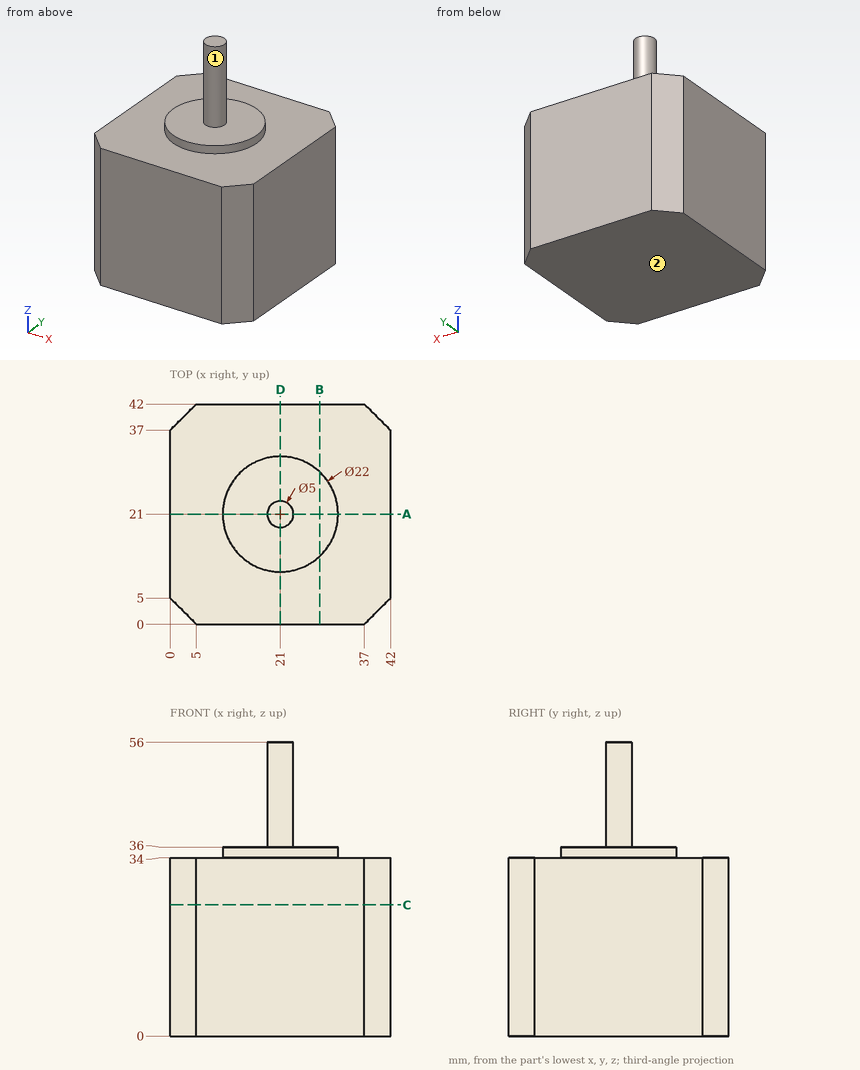
Study the drawing (mm; zero at the part's minimum x, y, z) and answer. A direction names the side the tool comes from. Give positions to 0.01 mm unless a question says otherwise; leave off trailing zeros. Write each loop counter-clockwise with the first axis right and the second up, starting at its lowest first coordinate (ties: lowest second). Pieces come first, ordered by that corner, then holes. Notation, with made-up numbers: (39, -0.75) -> (77, -0.75) arc R27 cw to (77, 31.25) -> close; hole circle Ø2 at (23.5, 23.25). An arc over 180 degrees is marked (long way). Answer as a JSON object with one key per item and string values. Group by question number.
1) Find section C-C (z = 25). Write down the section's boundary in (x, y), and give its area (3 significant figures).
2) Find section A-A (y = 21). Write down the section's boundary in (x, z).
3) Consider L1, parallel to Z at x = 31, y = 7; L2, parallel to Z at x = 25, y = 14.5. Determine where each line is inside the solid, lowest interval first. Write a range as from..to.
4) A tool of negligible diameter and unlimited length cuts with its end or side. For the marked faces 1 and 2, from which of +Z, -Z, +X, -X, +Y, -Y can it reach the whole face along a straight path? Write none if from no direction.
5) Find section B-B (x = 28.5). Write down the section's boundary in (y, z), and give its area (3 significant figures).
6) Each of these flat-tipped pins is pushed along its axis until it touches: P1, Ø6.5, axis at x = 23, y = 16, coming from the +Z side; P2, Ø5, axis at x = 14.5, y = 4.5, coming from the +Z side; P3, Ø1, axis at x = 29.5, y = 18.5, coming from the +Z side. Where does it stop, or does it pass through?
Values follow:
{
 "1": {"outline": "(0, 5) -> (5, 0) -> (37, 0) -> (42, 5) -> (42, 37) -> (37, 42) -> (5, 42) -> (0, 37) -> close", "area": "1,710 mm2"},
 "2": {"outline": "(0, 0) -> (42, 0) -> (42, 34) -> (32, 34) -> (32, 36) -> (23.5, 36) -> (23.5, 56) -> (18.5, 56) -> (18.5, 36) -> (10, 36) -> (10, 34) -> (0, 34) -> close"},
 "3": {"L1": "z = 0..34", "L2": "z = 0..36"},
 "4": {"face 1": "+Z", "face 2": "-Z, +X, -X, +Y, -Y"},
 "5": {"outline": "(0, 0) -> (42, 0) -> (42, 34) -> (29.05, 34) -> (29.05, 36) -> (12.95, 36) -> (12.95, 34) -> (0, 34) -> close", "area": "1,460 mm2"},
 "6": {"P1": "stops at z = 56", "P2": "stops at z = 34", "P3": "stops at z = 36"}
}
